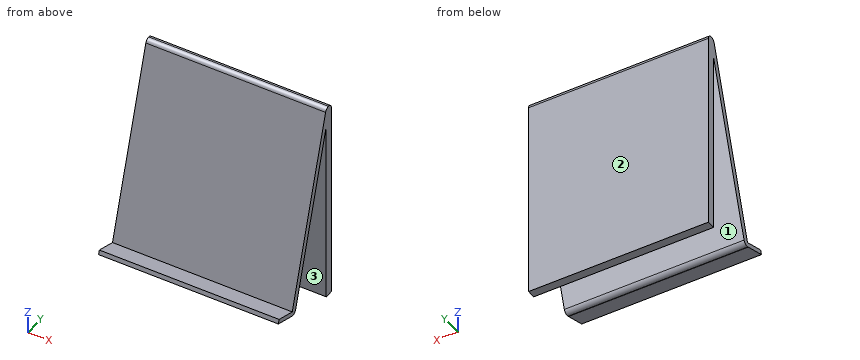
from build123d import *

# Parameters (mm, degrees)
F1_DEPTH      = 82.296
F1_DEPTH_BACK = 104.648
F2_R          = 5.08
F3_T1_DEPTH   = 205.8694200864
F4_R          = 5.08


# Not quite as in the source:
# - a fillet or chamfer that OpenCascade refuses, or shapes differently, is made with other operations: its cross-section is extruded or revolved along the edge and cut away or added


with BuildPart() as f1:
    # F0 (on Right) → F1 (new body, two sides)
    with BuildSketch(Plane.YZ) as f1_sk:
        Polygon((30.8638699353, 138.4397298098), (-26.3338502244, -53.1726228883), (-48.5219567113, -46.5493071791), (-49.8095880545, -50.8628719574), (-27.6214815676, -57.4861876667), (-22.003299054, -59.1632571598), (30.8638699353, 117.9417498623), (30.8638699353, -75.0317946076), (39.6366678178, -75.0317946076), (39.6366678178, 138.4397298098), align=None)
    extrude(amount=F1_DEPTH)
    extrude(f1_sk.sketch, amount=-F1_DEPTH_BACK)

    # F2
    f2_edges = [f1.edges().sort_by_distance(p)[0] for p in [
        (-11.176, 39.636668, 138.43973),
    ]]
    fillet(f2_edges, radius=F2_R)

    # F3: fillet of radius 5.08 on 1 edges, made by hand

    # F3_s2 → F3_t1 (cut)
    with BuildSketch(Plane.YZ.offset(-114.1107100432)):
        with BuildLine():
            ThreePointArc((34.6489539526, 138.4397298098), (31.6137560641, 137.4332999611), (29.7812013849, 134.8127903523))
            Line((29.7812013849, 134.8127903523), (30.8638699353, 138.4397298098))
            Line((30.8638699353, 138.4397298098), (34.6489539526, 138.4397298098))
        make_face()
    extrude(amount=F3_T1_DEPTH, mode=Mode.SUBTRACT)

    # F4
    f4_edges = [f1.edges().sort_by_distance(p)[0] for p in [
        (-11.176, -22.003299, -59.163257),
    ]]
    fillet(f4_edges, radius=F4_R)


solid = f1.part
Can you work these out from the model? Positions are in its coordinate system, mm. Face numbers are marked on the shaded views. Coordinates: 2 decimals unless noted, no trailing zeros. Loops run counter-clockwise (first coordinate to the right, second up) from the corner with the lowest first, then second, coordinate; pieces in that order, holes last. Notation, with made-up numbers: (49.5, -24.75) - (70.5, -24.75) arc R13 cw to (70.5, -15.75) - close; hole circle Ø4 at (23.25, 75.25). An arc over 180 degrees is marked (long way). Answer as a JSON object with one key per item and string values. Group by question number.
Item 1: For pin 1 (5 mm diameter, centred on x = -83, z = 6.5, fed in from -Y); pin 2 (6 mm diameter, centred on x = -36.5, z = 62, fed in from -Y); pin 3 (1.5 mm diameter, centred on x = -78.5, z = -37.5, fed in from -Y), each with a flat end and sliding along its axis, tell me the tip position at first contact or that it passes through.
Item 2: If we mould it in two halves opening along Y, with no side actions, what happens to the marked faces 1, 2 and 3? For each: released by +Y, released by -Y, zero draft, split by the parting line, or undercut.
Item 3: If we section it at C-C (y = -14): List the corners of the cut face in (x, z) for me.
Item 4: If I drill on L1, parallel to Y at x = -11.5, z = -3.5; L2, parallel to Y at x = -41, z = 58.5; L3, parallel to Y at x = -17, z = 121, over which ranges is the centre line in solid material (lowest first)? Write a range as from..to.
Item 5: If we section it at B-B (z = 92.5): List the corners of the cut face in (x, y) for me.
Item 6: If we section it at A-A (x = 71): List the corners of the cut face in (y, z) for me.
Returned:
{
 "1": {"pin 1": "stops at y = -9.27", "pin 2": "stops at y = 7.15", "pin 3": "stops at y = -21.88"},
 "2": {"face 1": "undercut", "face 2": "released by +Y", "face 3": "undercut"},
 "3": {"outline": "(-104.65, -32.35) - (82.3, -32.35) - (82.3, -11.85) - (-104.65, -11.85) - close"},
 "4": {"L1": "y = -11.51..-5.39, 30.86..39.64", "L2": "y = 7..13.12, 30.86..39.64", "L3": "y = 25.66..39.64"},
 "5": {"outline": "(-104.65, 17.15) - (82.3, 17.15) - (82.3, 23.27) - (-104.65, 23.27) - close; (-104.65, 30.86) - (82.3, 30.86) - (82.3, 39.64) - (-104.65, 39.64) - close"},
 "6": {"outline": "(-49.81, -50.86) - (-26.87, -57.71) arc R5.08 ccw to (-20.55, -54.3) - (30.86, 117.94) - (30.86, -75.03) - (39.64, -75.03) - (39.64, 133.36) arc R5.08 ccw to (34.6, 138.44) arc R5.08 ccw to (29.78, 134.81) - (-26.33, -53.17) - (-48.52, -46.55) - close"}
}
